Input: part model. Units: mm. Frame: model coordinates. Give positions to 0.01 mm unless a question says otherwise; leave off trailing zeros. Write each loop counter-clockwise with the first axis right and the second up, starting at its lowest first coordinate (ties: lowest second). Pieces come first, ordered by that corner, then holes. Notation, with made-up numbers: (21.25, 28) -> (77.25, 28) arc R12 ccw to (77.25, 44) -> close; hole circle Ø3 at (-32.75, 38.5). An arc over 180 degrees is marked (long way). Return JSON: item names as keys, results as strings. Group by question number.
Item 1: Section C-C, the plane x = -85.5. Return loops of the section in (y, z), then the cut area to 3 significant figures.
Item 2: Section A-A, the plane y = -20.5. Return loops of the section in (x, z).
Item 3: Section D-D, the plane z = 1.7. Count the separate pieces of the cut face and the enclosed holes in it, then the cut area to 3 significant figures.
Item 4: Line query: line 1 (Y direction, x = 85.5, z = 0.4); line 2 (Y direction, x = -28.5, z = 1.55); line 3 (Y direction, x = 74.5, z = 0.55). Output: solid intervals per line, ascending. Write a range as [from, to].
Item 5: Section B-B, the plane x = 85.5. Return loops of the section in (y, z).
Item 6: Pin query (flat end, axial travel): P1, Ø1, axis at y = 0, z = 1, coming from the +X side. Return the tip coordinate at first contact, or that it passes through.
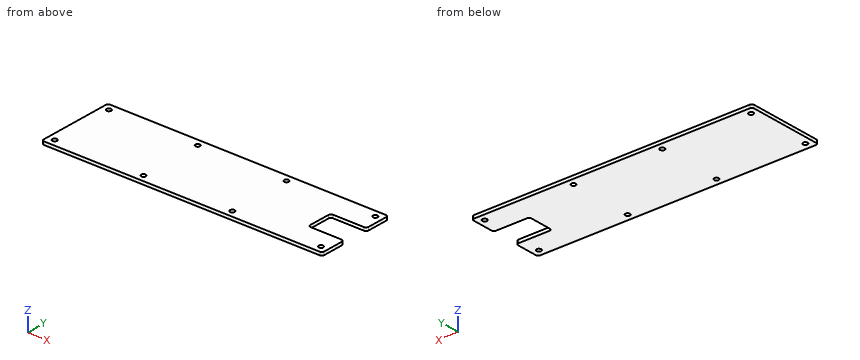
from build123d import *

# Parameters (mm, degrees)
F1_DEPTH = 2
F2_R     = 1.5
F3_DEPTH = 2.001


with BuildPart() as f1:
    # F0 (on Top) → F1 (new body)
    with BuildSketch(Plane.XY):
        with BuildLine():
            Line((88.5, 25), (-88.5, 25))
            ThreePointArc((-88.5, 25), (-89.56066, 24.56066), (-90, 23.5))
            Line((-90, 23.5), (-90, -23.5))
            ThreePointArc((-90, -23.5), (-89.56066, -24.56066), (-88.5, -25))
            Line((-88.5, -25), (88.5, -25))
            ThreePointArc((88.5, -25), (89.56066, -24.56066), (90, -23.5))
            Line((90, -23.5), (90, -10))
            ThreePointArc((90, -10), (89.56066, -8.93934), (88.5, -8.5))
            Line((88.5, -8.5), (68.5, -8.5))
            ThreePointArc((68.5, -8.5), (67.43934, -8.06066), (67, -7))
            Line((67, -7), (67, 7))
            ThreePointArc((67, 7), (67.43934, 8.06066), (68.5, 8.5))
            Line((68.5, 8.5), (88.5, 8.5))
            ThreePointArc((88.5, 8.5), (89.56066, 8.93934), (90, 10))
            Line((90, 10), (90, 23.5))
            ThreePointArc((90, 23.5), (89.56066, 24.56066), (88.5, 25))
        make_face()
    extrude(amount=F1_DEPTH)

    # F2 (on face) → F3 (cut, through all)
    with BuildSketch(Plane.XY.offset(2)):
        with Locations((-85.5, 20.5)):
            Circle(F2_R)
        with Locations((-85.5, -20.5)):
            Circle(F2_R)
        with Locations((-28.5, -20.5)):
            Circle(F2_R)
        with Locations((-28.5, 20.5)):
            Circle(F2_R)
        with Locations((28.5, -20.5)):
            Circle(F2_R)
        with Locations((28.5, 20.5)):
            Circle(F2_R)
        with Locations((85.5, -20.5)):
            Circle(F2_R)
        with Locations((85.5, 20.5)):
            Circle(F2_R)
    extrude(amount=-F3_DEPTH, mode=Mode.SUBTRACT)


solid = f1.part
Answer below:
{
 "1": {"outline": "(-25, 0) -> (-22, 0) -> (-22, 2) -> (-25, 2) -> close; (-19, 0) -> (19, 0) -> (19, 2) -> (-19, 2) -> close; (22, 0) -> (25, 0) -> (25, 2) -> (22, 2) -> close", "area": "88.0 mm2"},
 "2": {"outline": "(-90, 0) -> (-87, 0) -> (-87, 2) -> (-90, 2) -> close; (-84, 0) -> (-30, 0) -> (-30, 2) -> (-84, 2) -> close; (-27, 0) -> (27, 0) -> (27, 2) -> (-27, 2) -> close; (30, 0) -> (84, 0) -> (84, 2) -> (30, 2) -> close; (87, 0) -> (90, 0) -> (90, 2) -> (87, 2) -> close"},
 "3": {"separate pieces": "1", "enclosed holes": "8", "area": "8,550 mm2"},
 "4": {"line 1": "y = [-25, -22], [-19, -8.5], [8.5, 19], [22, 25]", "line 2": "y = [-25, -22], [-19, 19], [22, 25]", "line 3": "y = [-25, -8.5], [8.5, 25]"},
 "5": {"outline": "(-25, 0) -> (-22, 0) -> (-22, 2) -> (-25, 2) -> close; (-19, 0) -> (-8.5, 0) -> (-8.5, 2) -> (-19, 2) -> close; (8.5, 0) -> (19, 0) -> (19, 2) -> (8.5, 2) -> close; (22, 0) -> (25, 0) -> (25, 2) -> (22, 2) -> close"},
 "6": {"P1": "stops at x = 67"}
}
